from build123d import *

# Parameters (mm, degrees)
F0_W     = 40
F0_H     = 3
F0_W_2   = 3
F0_H_2   = 40
F1_DEPTH = 3


with BuildPart() as f1:
    # F0 (on Top) → F1 (new body)
    with BuildSketch(Plane.XY):
        Polygon((85, 75), (85, 105), (65, 105), (25, 105), (-25, 105), (-65, 105), (-85, 105), (-85, 75), (-85, 35), (-85, -35), (-85, -75), (-85, -105), (-65, -105), (-25, -105), (25, -105), (65, -105), (85, -105), (85, -75), (85, -35), (85, 35), align=None)
        with Locations((45, 106.5)):
            Rectangle(F0_W, F0_H)
        with Locations((86.5, 55)):
            Rectangle(F0_W_2, F0_H_2)
        with Locations((-45, 106.5)):
            Rectangle(F0_W, F0_H)
        with Locations((86.5, -55)):
            Rectangle(F0_W_2, F0_H_2)
        with Locations((-86.5, 55)):
            Rectangle(F0_W_2, F0_H_2)
        with Locations((45, -106.5)):
            Rectangle(F0_W, F0_H)
        with Locations((-86.5, -55)):
            Rectangle(F0_W_2, F0_H_2)
        with Locations((-45, -106.5)):
            Rectangle(F0_W, F0_H)
    extrude(amount=F1_DEPTH)


solid = f1.part
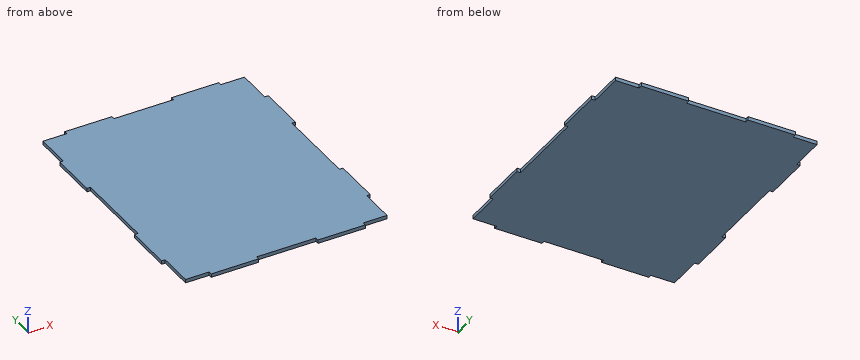
Geometry check sheet. Reference: the model listing, model coordinates, mm. Round coordinates to 2 decimals unless told otherwise and drop trailing zeros. Loops run counter-clockwise (first coordinate to the right, second up) from the corner with the lowest first, then second, coordinate; pieces in that order, holes last.
Item 1: Gauge pin test, flat ends, axial feed: pin 1 (0.9 mm diameter, centred on y = -4.5, z = 2, fed in from -X); pin 2 (1.5 mm diameter, centred on x = -86.5, z = 1, fed in from +Y); pin 3 (0.9 mm diameter, centred on x = 78, z = 1.5, fed in from -Y). Record the tip position at first contact, or that the pin passes through.
Item 2: Cross-section at A-A on y = 23. Record the boundary of the cut face in (x, z).
Item 3: Cross-section at B-B on x = -7. Record the boundary of the cut face in (y, z).
Item 4: Thickness scan on line 1 (Y direction, x = 78, z = 2.1); line 2 (X direction, y = 13, z = 2.8). Record the ranges inside material, lowest first.
Answer sheet:
1. pin 1: stops at x = -85
1. pin 2: stops at y = 75
1. pin 3: stops at y = -105
2. outline: (-85, 0) - (85, 0) - (85, 3) - (-85, 3) - close
3. outline: (-105, 0) - (105, 0) - (105, 3) - (-105, 3) - close
4. line 1: y = -105 to 105
4. line 2: x = -85 to 85
